from build123d import *

# Parameters (mm, degrees)
CROQUIS1_W              = 100
CROQUIS1_H              = 24
CROQUIS1_R              = 2.017504942
CROQUIS1_R_2            = 2.25
SALIENTE_EXTRUIR1_DEPTH = 5
CROQUIS2_R              = 2.5
CORTAR_EXTRUIR1_DEPTH   = 2
CORTAR_EXTRUIR5_DEPTH   = 141


with BuildPart() as part:
    # Croquis1 → Saliente-Extruir1 (new body)
    with BuildSketch(Plane(origin=(0, 0, 0), x_dir=(1, 0, 0), z_dir=(0, 1, 0))):
        Rectangle(CROQUIS1_W, CROQUIS1_H)
        with Locations(Location((-47, -9, 0), (0, 0, 270))):
            Circle(CROQUIS1_R, mode=Mode.SUBTRACT)
        with Locations(Location((-40, -7, 0), (0, 0, 270))):
            Circle(CROQUIS1_R_2, mode=Mode.SUBTRACT)
        with Locations(Location((40, -7, 0), (0, 0, 270))):
            Circle(CROQUIS1_R_2, mode=Mode.SUBTRACT)
        with Locations(Location((47, -9, 0), (0, 0, 270))):
            Circle(CROQUIS1_R, mode=Mode.SUBTRACT)
    extrude(amount=SALIENTE_EXTRUIR1_DEPTH)

    # Croquis2 → Cortar-Extruir1 (cut)
    # profile 1 of 2: a face of its own
    with BuildSketch(Plane(origin=(0, 5, 0), x_dir=(1, 0, 0), z_dir=(0, 1, 0))):
        with BuildLine():
            Line((-44, -3), (-44, -12))
            Line((-44, -12), (-36, -12))
            Line((-36, -12), (-36, -3))
            ThreePointArc((-36, -3), (-36.878679656, -0.878679656), (-39, 0))
            Line((-39, 0), (-41, 0))
            ThreePointArc((-41, 0), (-43.121320344, -0.878679656), (-44, -3))
        make_face()
        with Locations(Location((-40, -7, 0), (0, 0, 270))):
            Circle(CROQUIS2_R, mode=Mode.SUBTRACT)
    # profile 2 of 2: a face of its own
    with BuildSketch(Plane(origin=(0, 5, 0), x_dir=(1, 0, 0), z_dir=(0, 1, 0))):
        with BuildLine():
            Line((41, 0), (39, 0))
            ThreePointArc((39, 0), (36.878679656, -0.878679656), (36, -3))
            Line((36, -3), (36, -12))
            Line((36, -12), (44, -12))
            Line((44, -12), (44, -3))
            ThreePointArc((44, -3), (43.121320344, -0.878679656), (41, 0))
        make_face()
    extrude(amount=-CORTAR_EXTRUIR1_DEPTH, mode=Mode.SUBTRACT)

    # Croquis3 → Cortar-Extruir5 (cut)
    with BuildSketch(Plane.ZY.offset(50)):
        Polygon((-12, 5), (-12, 0.2), (-6.100895765, 3.605849418), (-3.686156124, 5), align=None)
        Polygon((-12.757171087, 0.2), (-12, 0.2), (-12, 5), (-3.686156124, 5), (-3.039853353, 5.373143079), (-12.757171087, 5.373143079), align=None)
    extrude(amount=-CORTAR_EXTRUIR5_DEPTH, mode=Mode.SUBTRACT)


solid = part.part
Geometry: final body of the model. Coordinates: model frame, mm. A direction names the side the tool comes from. Give positions to 0.01 mm unless a question says otherwise; leave off trailing zeros. Order: outer loops, then holes, each group sorted by start corner. A loop starts at its lowest first (then second) coordinate and runs counter-clockwise, first axis right, second up. Notation, with made-up numbers: (5, -13.75) -> (9, -13.75) arc R27 ccw to (9, 16.25) -> close; hole circle Ø10 at (23, 78.5). An arc over 180 degrees is marked (long way). Put each result on its own line as item: value.
Q1. Reachability of faces 4 (the face through (-42.44, 4.01, 6.46)), 5 (the face through (-50, 2, 3)), 6 (the face through (-44, 4, 7)) from +Z, -Z, +X, -X, +Y, -Y: full face, straight path, thin tool, end or side. Return the list, or none.
Here are the results:
face 4: +Y
face 5: +Z, -Z, -X, +Y, -Y
face 6: +Z, +Y
Q2. Section C-C, the plane x = -47. Return loops of the section in (y, z), then the cut area to 3 significant figures.
Here are the results:
outline: (0, -12) -> (0.2, -12) -> (5, -3.69) -> (5, 6.98) -> (0, 6.98) -> close; (0, 11.02) -> (5, 11.02) -> (5, 12) -> (0, 12) -> close
area: 79.9 mm^2
Q3. Material intervals for L1, parallel to X at y = 2.5, z = 8; L2, parallel to X at y = 4, z = 10.75; L3, parallel to Z at x = 40, y = 1.45, sorted ascending.
Here are the results:
L1: x = -50 to -48.75, -45.25 to -42.02, -37.98 to 37.98, 42.02 to 45.25, 48.75 to 50
L2: x = -50 to -48, -46 to -44, -36 to 36, 44 to 46, 48 to 50
L3: z = -9.83 to 4.75, 9.25 to 12
Q4. Pin query (flat end, axial travel): pin 1 (1 mm diameter, centred on x = -39.5, y = 4.5, fed in from +Z); pin 2 (5 mm diameter, centred on x = 40, z = 7, fed in from +Y). Return the tip coordinate at first contact, or that it passes through.
Here are the results:
pin 1: stops at z = 9.5
pin 2: stops at y = 3
Q5. Section A-A, the plane x = 40. Return loops of the section in (y, z), then the cut area to 3 significant figures.
Here are the results:
outline: (0, -12) -> (0.2, -12) -> (5, -3.69) -> (5, 0) -> (3, 0) -> (3, 4.75) -> (0, 4.75) -> close; (0, 9.25) -> (3, 9.25) -> (3, 12) -> (0, 12) -> close
area: 62.5 mm^2
Q6. Section B-B, the plane y = 1.6. Count the separate pieces of the cut face and the enclosed holes in it, then the cut area to 3 significant figures.
Here are the results:
separate pieces: 1
enclosed holes: 4
area: 2,100 mm^2
Q7. Section D-D, the plane x = -2.5. Return loops of the section in (y, z).
Here are the results:
outline: (0, -12) -> (0.2, -12) -> (5, -3.69) -> (5, 12) -> (0, 12) -> close
Q8. Draft query along Z for faces 1 (the face through (-36, 4, 8)), 2 (the face through (40, 4, 0)), 3 (the face through (-42, 3, 5)). Return one class per face: released by +Z, released by -Z, zero draft, split by the parting line, or undercut.
Here are the results:
face 1: zero draft
face 2: released by +Z
face 3: undercut
